```python
from build123d import *

# Parameters (mm, degrees)
F0_W     = 57
F0_H     = 13
F1_DEPTH = 13
F2_W     = 57
F2_H     = 13
F2_R     = 0.75
F3_DEPTH = 1.6
F4_ANGLE = -180
F5_ANGLE = -180
F6_R     = 0.75
F7_DEPTH = 5


with BuildPart() as f1:
    # F0 (on Top) → F1 (new body)
    with BuildSketch(Plane.XY):
        Rectangle(F0_W, F0_H)
    extrude(amount=F1_DEPTH)

    # F2 (on face) → F3 (cut)
    with BuildSketch(Plane.XY.offset(13)):
        Rectangle(F2_W, F2_H)
        with BuildLine():
            ThreePointArc((-6.027774, 3.5), (-5.005, 0), (-6.027774, -3.5))
            Line((-6.027774, -3.5), (-16.982226, -3.5))
            ThreePointArc((-16.982226, -3.5), (-18.005, 0), (-16.982226, 3.5))
            Line((-16.982226, 3.5), (-6.027774, 3.5))
        make_face(mode=Mode.SUBTRACT)
        with BuildLine():
            ThreePointArc((6.017774, -3.5), (4.995, 0), (6.017774, 3.5))
            Line((6.017774, 3.5), (16.972226, 3.5))
            ThreePointArc((16.972226, 3.5), (17.995, 0), (16.972226, -3.5))
            Line((16.972226, -3.5), (6.017774, -3.5))
        make_face(mode=Mode.SUBTRACT)
        with Locations((-17.13, 0)):
            Circle(F2_R)
        with Locations((-5.88, 0)):
            Circle(F2_R)
        with Locations((5.87, 0)):
            Circle(F2_R)
        with Locations((17.12, 0)):
            Circle(F2_R)
    extrude(amount=-F3_DEPTH, mode=Mode.SUBTRACT)


with BuildPart() as f1_1:
    # F4: moved
    add(f1.part.rotate(Axis((0, 6.5, 0), (1, 0, 0)), F4_ANGLE))


with BuildPart() as f1_2:
    # F5: moved
    add(f1_1.part.rotate(Axis((0, 6.5, 0), (1, 0, 0)), F5_ANGLE))

    # F6 (on face) → F7 (cut)
    with BuildSketch(Plane.XY.offset(11.4)):
        Circle(F6_R)
    extrude(amount=-F7_DEPTH, mode=Mode.SUBTRACT)


solid = f1_2.part
```
Model file for the job. Use its own axes, mm. A direction names the side the tool comes from. Coordinates: 2 decimals unless noted, no trailing zeros. Order: outer loops, then holes, each group sorted by start corner. A loop starts at its lowest first (then second) coordinate and runs counter-clockwise, first axis right, second up. Notation, with made-up numbers: M 38.5,10 L 89.5,10 A12 cw 89.5,18 Z; hole C 84.25,60 d3. An arc over 180 degrees is marked long. Answer as CSV lines item,"result".
(1) 3-axis set-ups, long thin cutter, end or side, ignore diameter. For faces 4 (the flat face through (11, 3.5, 12)), 5 (the cylindrical face through (-0.75, 0.03, 8.94)), 6 (the flat face through (28.5, 0, 6)), 7 (the flat face through (12, -3.5, 12)): which of +Z, -Z, +X, -X, +Y, -Y reach the whole face in a straight line?
Geometry says:
face 4,"+Z, +X, -X, +Y"
face 5,"+Z"
face 6,"+Z, -Z, +X, +Y, -Y"
face 7,"+Z, +X, -X, -Y"
(2) Band-saw the part on A-A, the plane x = 0. List the corners of the cut face in (y, z).
Geometry says:
outline,"M -6.5,0 L 6.5,0 L 6.5,11.4 L 0.75,11.4 L 0.75,6.4 L -0.75,6.4 L -0.75,11.4 L -6.5,11.4 Z"
(3) Pull direction X, two halves, no side cores. Call faces 1 (the flat face through (-28.5, 0, 6)), 2 (the flat face through (0, 6.5, 6)), 3 (the flat face through (0, 0, 6.4)): +X half, -X half, draft (parallel to the pull), parting line (faces both ways), or undercut.
Geometry says:
face 1,"-X half"
face 2,"draft"
face 3,"undercut"
(4) Wall check: line 1 along Y through (x, z) = (-17.13, 12.55); line 2 along Z through (x, y) = (-20, -2.5); line 3 along Y through (x, z) = (16, 12). Give the ranges that are in metal, low to high.
Geometry says:
line 1,"y = -3.26 to -0.75, 0.75 to 3.26"
line 2,"z = 0 to 11.4"
line 3,"y = -3.5 to 3.5"
(5) Band-saw the part on C-C, the plane x = -8.5. List the corners of the cut face in (y, z).
Geometry says:
outline,"M -6.5,0 L 6.5,0 L 6.5,11.4 L 3.5,11.4 L 3.5,13 L -3.5,13 L -3.5,11.4 L -6.5,11.4 Z"
(6) Flat gauge pins, fed straight in: pin 1 (1.4 mm diameter, centred on x = -17.13, y = 0, fed in from +Z); pin 2 (1.8 mm diameter, centred on x = 13.5, z = 12.5, fed in from -Y); pin 3 (1.8 mm diameter, centred on x = -13.5, z = 12.5, fed in from +Y). Where does each tip first touch, or does it go through?
Geometry says:
pin 1,"stops at z = 11.4"
pin 2,"stops at y = -3.5"
pin 3,"stops at y = 3.5"
(7) Band-saw the part on D-D, the plane y = 5.75. List the corners of the cut face in (x, z).
Geometry says:
outline,"M -28.5,0 L 28.5,0 L 28.5,11.4 L -28.5,11.4 Z"
